Read the model definition and answer for the solid it produces. Units are mm, in the model's axes. A direction names the side the tool comes from. Coordinates: 2 decimals unless noted, no trailing zeros. Order: outer loops, then holes, each group sorted by start corner. A loop starts at its lowest first (then second) coordinate and runs counter-clockwise, first axis right, second up. Notation, with made-up numbers: M -17,50 L 30,50 A13 ccw 30,71 Z; hole C -38.5,48.25 d9. An arc over 180 degrees is marked long. One line per question, with ' | ' between items. Start each with the question number.
1) Find section B-B, the plane z = 0. Write down the section's boundary in (x, y).
2) Find section A-A, the plane y = 10. Write down the section's boundary in (x, z).
3) Consider probe 1 along Y at (x, z) = (17.5, -6); probe 2 along X at (y, z) = (38, 20.5). Determine where each line is inside the solid, lowest interval first.
4) Find section C-C, the plane x = 30. Write down the section's boundary in (y, z), plus the area to 3 significant figures.
5) Find section D-D, the plane z = -9.5. Write down the section's boundary in (x, y).
6) The mould has two halves that part along X. Classify faces 4 (the face through (-8, 6, -11.25)), 5 (the face through (31.69, -0.36, -13.09)), 6 (the face through (-8.237, 27, 0)): +X half, -X half, draft (parallel to the pull), parting line (faces both ways), or undercut.
7) Given P1, Ø8, axis at y = 42.5, z = 18, coming from the +X side; P2, Ø6.5, axis at x = -3, y = 12.5, coming from the -Z side; P3, Ø1.5, axis at x = 18, z = -4, coming from the +Y side, each flat-ended and moving along its own axis, determine where each tip first touches the part or whether it passes through.
8) A tool of negligible diameter and unlimited length cuts with its end or side. For faces 1 (the face through (-8, 6, 11.25)), 2 (the face through (17, 0, 0)), 3 (the face through (-7.873, 54.732, -0.495)), from which of +Z, -Z, +X, -X, +Y, -Y can it reach the whole face along a straight path? Write none if from no direction.
from build123d import *

# Parameters (mm, degrees)
SKETCH1_R                  = 2.5
SKETCH1_W                  = 25
SKETCH1_H                  = 22.5
BASE_FLANGE3_DEPTH         = 0.7366
SKETCHED_START             = -22.5
SKETCHED_BEND1_DEPTH       = 45
SKETCHED_BEND1_2_DEPTH     = 11.25
SKETCHED_START_2           = 11.25
SKETCHED_BEND1_3_DEPTH     = 11.25
SKETCHED_START_3           = -63
SKETCHED_BEND1_4_OUTLINE_W = 0.7366
SKETCHED_BEND1_4_OUTLINE_H = 45
SKETCHED_BEND1_4_DEPTH     = 38
SKETCHED_START_4           = -8.2366
SKETCHED_BEND1_5_DEPTH     = 0.7366


with BuildPart() as part:
    # Base-Flange3: sheet metal written as solids
    # Sketch1 → Base-Flange3 (new body)
    with BuildSketch(Plane(origin=(0, 0, 0), x_dir=(1, 0, 0), z_dir=(0, 1, 0))):
        with BuildLine():
            Line((-40, 22.5), (40, 22.5))
            Line((40, 22.5), (40, -22.5))
            Line((40, -22.5), (-40, -22.5))
            ThreePointArc((-40, -22.5), (-62.5, 0), (-40, 22.5))
        make_face()
        with Locations(Location((10, -11.25, 0), (0, 0, 270))):
            Circle(SKETCH1_R, mode=Mode.SUBTRACT)
        with Locations(Location((10, 11.25, 0), (0, 0, 270))):
            Circle(SKETCH1_R, mode=Mode.SUBTRACT)
        with Locations(Location((30, -11.25, 0), (0, 0, 270))):
            Circle(SKETCH1_R, mode=Mode.SUBTRACT)
        with Locations(Location((30, 11.25, 0), (0, 0, 270))):
            Circle(SKETCH1_R, mode=Mode.SUBTRACT)
        with Locations((-12.5, 0)):
            Rectangle(SKETCH1_W, SKETCH1_H, mode=Mode.SUBTRACT)
    extrude(amount=-BASE_FLANGE3_DEPTH)

    # Sketched Bend1: read off the stored shape, not the designer's step
    # Sketched Bend1 outline → Sketched Bend1 (cut)
    with BuildSketch(Plane.XY.offset(SKETCHED_START)):
        with BuildLine():
            ThreePointArc((-6.7634, -0.7366), (-7.5, -0.539228625), (-8.039228625, 0))
            Line((-8.039228625, 0), (-25, 0))
            Line((-25, 0), (-25, -0.7366))
            Line((-25, -0.7366), (-6.7634, -0.7366))
        make_face()
    extrude(amount=SKETCHED_BEND1_DEPTH, mode=Mode.SUBTRACT)

    # Sketched Bend1 2 outline → Sketched Bend1 2 (add)
    with BuildSketch(Plane.XY.offset(SKETCHED_START)):
        with BuildLine():
            Line((-7.5, 17.237627139), (-8.2366, 17.237627139))
            Line((-8.2366, 17.237627139), (-8.2366, 0.7366))
            ThreePointArc((-8.2366, 0.7366), (-8.186401927, 0.355307783), (-8.039228625, 0))
            Line((-8.039228625, 0), (-6.7634, 0))
            ThreePointArc((-6.7634, 0), (-7.284254855, 0.215745145), (-7.5, 0.7366))
            Line((-7.5, 0.7366), (-7.5, 17.237627139))
        make_face()
    extrude(amount=SKETCHED_BEND1_2_DEPTH)

    # Sketched Bend1 3 outline → Sketched Bend1 3 (add)
    with BuildSketch(Plane.XY.offset(SKETCHED_START_2)):
        with BuildLine():
            Line((-7.5, 17.237627139), (-8.2366, 17.237627139))
            Line((-8.2366, 17.237627139), (-8.2366, 0.7366))
            ThreePointArc((-8.2366, 0.7366), (-8.186401927, 0.355307783), (-8.039228625, 0))
            Line((-8.039228625, 0), (-6.7634, 0))
            ThreePointArc((-6.7634, 0), (-7.284254855, 0.215745145), (-7.5, 0.7366))
            Line((-7.5, 0.7366), (-7.5, 17.237627139))
        make_face()
    extrude(amount=SKETCHED_BEND1_3_DEPTH)

    # Sketched Bend1 4 outline → Sketched Bend1 4 (cut)
    with BuildSketch(Plane.YZ.offset(SKETCHED_START_3)):
        with Locations((-0.3683, 0)):
            Rectangle(SKETCHED_BEND1_4_OUTLINE_W, SKETCHED_BEND1_4_OUTLINE_H)
    extrude(amount=SKETCHED_BEND1_4_DEPTH, mode=Mode.SUBTRACT)

    # Sketched Bend1 5 outline → Sketched Bend1 5 (add)
    with BuildSketch(Plane.YZ.offset(SKETCHED_START_4)):
        with BuildLine():
            ThreePointArc((32.237627139, -22.5), (54.737627139, 0), (32.237627139, 22.5))
            Line((32.237627139, 22.5), (17.237627139, 22.5))
            Line((17.237627139, 22.5), (17.237627139, -22.5))
            Line((17.237627139, -22.5), (32.237627139, -22.5))
        make_face()
    extrude(amount=SKETCHED_BEND1_5_DEPTH)


solid = part.part
Report:
1) outline: M -8.24,17.24 L -7.5,17.24 L -7.5,54.74 L -8.24,54.74 Z; M 0,-0.74 L 40,-0.74 L 40,0 L 0,0 Z
2) outline: M -8.24,-22.5 L -7.5,-22.5 L -7.5,-11.25 L -8.24,-11.25 Z; M -8.24,11.25 L -7.5,11.25 L -7.5,22.5 L -8.24,22.5 Z
3) probe 1: y = -0.74 to 0 | probe 2: x = -8.24 to -7.5
4) outline: M -0.74,-22.5 L 0,-22.5 L 0,-13.75 L -0.74,-13.75 Z; M -0.74,-8.75 L 0,-8.75 L 0,8.75 L -0.74,8.75 Z; M -0.74,13.75 L 0,13.75 L 0,22.5 L -0.74,22.5 Z | area: 25.8 mm^2
5) outline: M -8.24,17.24 L -7.5,17.24 L -7.5,52.63 L -8.24,52.63 Z; M 0,-0.74 L 8.21,-0.74 L 8.21,0 L 0,0 Z; M 11.79,-0.74 L 28.21,-0.74 L 28.21,0 L 11.79,0 Z; M 31.79,-0.74 L 40,-0.74 L 40,0 L 31.79,0 Z
6) face 4: draft | face 5: undercut | face 6: -X half
7) P1: stops at x = -7.5 | P2: passes through | P3: stops at y = 0
8) face 1: -X, -Y | face 2: +Z, -Z, +X, +Y | face 3: +X, -X, +Y
